Verification items for the finished model (mm, model axes). Face numbers are marked on the shaded views. A direction names the side the tool comes from. Give positions to 0.01 mm unless a question says otherwise; leave off trailing zeros. Order: outer loops, then holes, each group sorted by start corner. A loop starts at its lowest first (then second) coordinate and runs counter-clockwise, first axis right, second up.
from build123d import *

# Parameters (mm, degrees)
SZKIC1_R                    = 11
SZKIC1_R_2                  = 4
DODANIE_WYCI_GNI_CIE1_DEPTH = 30
SZKIC5_W                    = 15
SZKIC5_H                    = 7
DODANIE_WYCI_GNI_CIE2_DEPTH = 30
SZKIC6_W                    = 15
SZKIC6_H                    = 7
DODANIE_WYCI_GNI_CIE3_DEPTH = 30
SZKIC7_W                    = 7.450165565
SZKIC7_H                    = 12
DODANIE_WYCI_GNI_CIE4_DEPTH = 30
WYTNIJ_WYCI_GNI_CIE1_REACH  = 42.112
SZKIC8_R                    = 2


with BuildPart() as part:
    # Szkic1 → Dodanie-wyciągnięcie1 (new body)
    with BuildSketch(Plane.XY):
        Circle(SZKIC1_R)
        Circle(SZKIC1_R_2, mode=Mode.SUBTRACT)
    extrude(amount=DODANIE_WYCI_GNI_CIE1_DEPTH)

    # Szkic5 → Dodanie-wyciągnięcie2 (add)
    with BuildSketch(Plane(origin=(0, 0, 0), x_dir=(-1, 0, 0), z_dir=(0, 0, -1))):
        with Locations((7.5, -7.5)):
            Rectangle(SZKIC5_W, SZKIC5_H)
    extrude(amount=-DODANIE_WYCI_GNI_CIE2_DEPTH)

    # Szkic6 → Dodanie-wyciągnięcie3 (add)
    with BuildSketch(Plane.XY):
        with Locations((7.5, -7.5)):
            Rectangle(SZKIC6_W, SZKIC6_H)
    extrude(amount=DODANIE_WYCI_GNI_CIE3_DEPTH)

    # Szkic7 → Dodanie-wyciągnięcie4 (add)
    with BuildSketch(Plane.XY):
        with Locations((11.274917218, 2)):
            Rectangle(SZKIC7_W, SZKIC7_H)
        with Locations((-11.274917218, 2)):
            Rectangle(SZKIC7_W, SZKIC7_H)
    extrude(amount=DODANIE_WYCI_GNI_CIE4_DEPTH)

    # Szkic8 → Wytnij-wyciągnięcie1 (cut, up to next)
    with BuildSketch(Plane.XZ.offset(11), mode=Mode.PRIVATE) as wytnij_wyci_gni_cie1_sk1:
        with Locations(Location((-12, 24, 0), (0, 0, 270))):
            Circle(SZKIC8_R)
    wytnij_wyci_gni_cie1_tool1 = extrude(wytnij_wyci_gni_cie1_sk1.sketch, amount=-WYTNIJ_WYCI_GNI_CIE1_REACH, mode=Mode.PRIVATE) & part.part
    # Szkic8 → Wytnij-wyciągnięcie1 (cut, up to next)
    with BuildSketch(Plane.XZ.offset(11), mode=Mode.PRIVATE) as wytnij_wyci_gni_cie1_sk2:
        with Locations(Location((12, 24, 0), (0, 0, 270))):
            Circle(SZKIC8_R)
    wytnij_wyci_gni_cie1_tool2 = extrude(wytnij_wyci_gni_cie1_sk2.sketch, amount=-WYTNIJ_WYCI_GNI_CIE1_REACH, mode=Mode.PRIVATE) & part.part
    # Szkic8 → Wytnij-wyciągnięcie1 (cut, up to next)
    with BuildSketch(Plane.XZ.offset(11), mode=Mode.PRIVATE) as wytnij_wyci_gni_cie1_sk3:
        with Locations(Location((12, 6, 0), (0, 0, 270))):
            Circle(SZKIC8_R)
    wytnij_wyci_gni_cie1_tool3 = extrude(wytnij_wyci_gni_cie1_sk3.sketch, amount=-WYTNIJ_WYCI_GNI_CIE1_REACH, mode=Mode.PRIVATE) & part.part
    # Szkic8 → Wytnij-wyciągnięcie1 (cut, up to next)
    with BuildSketch(Plane.XZ.offset(11), mode=Mode.PRIVATE) as wytnij_wyci_gni_cie1_sk4:
        with Locations(Location((-12, 6, 0), (0, 0, 270))):
            Circle(SZKIC8_R)
    wytnij_wyci_gni_cie1_tool4 = extrude(wytnij_wyci_gni_cie1_sk4.sketch, amount=-WYTNIJ_WYCI_GNI_CIE1_REACH, mode=Mode.PRIVATE) & part.part
    add(wytnij_wyci_gni_cie1_tool1.solids().sort_by_distance((-12, -11, 24))[0], mode=Mode.SUBTRACT)
    add(wytnij_wyci_gni_cie1_tool2.solids().sort_by_distance((12, -11, 24))[0], mode=Mode.SUBTRACT)
    add(wytnij_wyci_gni_cie1_tool3.solids().sort_by_distance((12, -11, 6))[0], mode=Mode.SUBTRACT)
    add(wytnij_wyci_gni_cie1_tool4.solids().sort_by_distance((-12, -11, 6))[0], mode=Mode.SUBTRACT)


solid = part.part
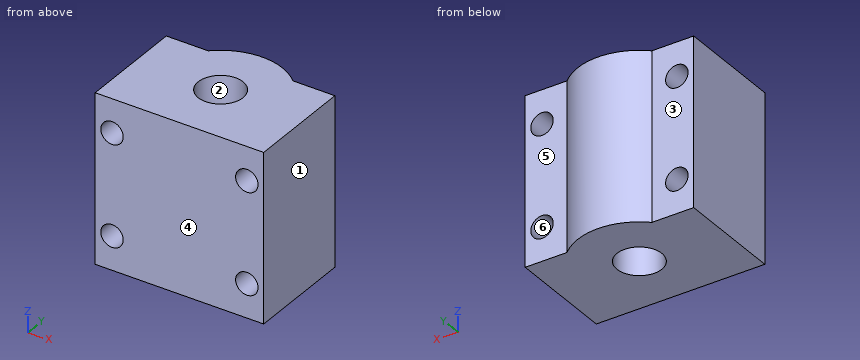
(1) Release check for a two-part mould opening along Y. For the marked faces 1, 2, 3 and 4 record: pulls with the +Y half, pulls with the -Y half, needs draft (parallel to the pull), parting line crosses it, or undercut.
Solved:
face 1: needs draft
face 2: undercut
face 3: pulls with the +Y half
face 4: pulls with the -Y half
(2) Section check A-A, the plane z = 6. Enter the section's corners in (x, y).
Solved:
outline: (-15, -11) - (-14, -11) - (-14, 8) - (-15, 8) - close; (-10, -11) - (10, -11) - (10, 8) - (7.55, 8) arc R11 ccw to (-7.55, 8) - (-10, 8) - close; (14, -11) - (15, -11) - (15, 8) - (14, 8) - close; hole circle Ø8 at (0, 0)
(3) Section check B-B, the plane y = 0. Enter the section's corners in (x, z), then the cut area to 3 significant figures.
Solved:
outline: (-15, 0) - (-4, 0) - (-4, 30) - (-15, 30) - close; (4, 0) - (15, 0) - (15, 30) - (4, 30) - close; hole circle Ø4 at (-12, 6); hole circle Ø4 at (-12, 24); hole circle Ø4 at (12, 6); hole circle Ø4 at (12, 24)
area: 610 mm2
(4) Set-up check for the marked faces 5 and 6: record each of +Z, -Z, +X, -X, +Y, -Y from which the full face is reachable in a straight line by a thin tool's end or side.
Solved:
face 5: +Z, -Z, +X, +Y
face 6: +Y, -Y
(5) Go/stop test with flat-tipped pins: pin 1 (1.5 mm diameter, centred on x = 4, z = 7, fed in from +Y); pin 2 (8 mm diameter, centred on x = 10.5, z = 18.5, fed in from +Y); pin 3 (2.5 mm diameter, centred on x = 12, z = 24, fed in from -Y); pin 4 (12 mm diameter, centred on x = 11, z = 8, fed in from +Y). Record where each tip stops, or that it passes through.
Solved:
pin 1: stops at y = 10.51
pin 2: stops at y = 8.87
pin 3: passes through
pin 4: stops at y = 9.8
(6) Scan lines: line 1 (X direction, y = -6.75, z = 6); line 2 (Z direction, x = -12.5, y = -4); line 3 (X direction, y = 0.25, z = 16.75). Record each from-to range of solid material in increasing order.
Solved:
line 1: x = -15 to -14, -10 to 10, 14 to 15
line 2: z = 0 to 4.06, 7.94 to 22.06, 25.94 to 30
line 3: x = -15 to -3.99, 3.99 to 15
(7) Section check D-D, the plane y = -6. Enter the section's corners in (x, z), then the cut area to 3 significant figures.
Solved:
outline: (-15, 0) - (15, 0) - (15, 30) - (-15, 30) - close; hole circle Ø4 at (-12, 6); hole circle Ø4 at (-12, 24); hole circle Ø4 at (12, 6); hole circle Ø4 at (12, 24)
area: 850 mm2
(8) Section check C-C, the plane x = -2. Enter the section's corners in (y, z).
Solved:
outline: (-11, 0) - (-3.46, 0) - (-3.46, 30) - (-11, 30) - close; (3.46, 0) - (10.82, 0) - (10.82, 30) - (3.46, 30) - close
